Part model, mm, in its own coordinate system. Face numbers are marked on the shaded views. A direction names the side the tool comes from. Give positions to 0.01 mm unless a question says otherwise; leave off trailing zeros. Order: outer loops, then holes, each group sorted by start corner. A loop starts at its lowest first (then second) coordinate and runs counter-clockwise, first axis right, second up. Notation, with made-up numbers: M -35.5,71.5 L -18.5,71.5 A15 cw -18.5,97.5 Z; hole C 7,49.5 d2. An arc over 180 degrees is marked long. Write each question's results on one line, items separated by ' | '. Start each with the question number.
from build123d import *

# Parameters (mm, degrees)
SKETCH_1_R               = 222
EXTRUDE_1_DEPTH          = 76.4
EXTRUDE_2_DEPTH          = 76.4
CUT_EXTRUDE_1_DEPTH      = 508.563749691
CUT_EXTRUDE_1_DEPTH_BACK = 508.563749691
SKETCH_3_R               = 220.4
CUT_EXTRUDE_2_DEPTH      = 508.563749691
CUT_EXTRUDE_2_DEPTH_BACK = 508.563749691
SKETCH_5_R               = 222
EXTRUDE_3_DEPTH          = 1.6
EXTRUDE_4_DEPTH          = 1.6
CUT_EXTRUDE_3_DEPTH      = 508.807049971
CUT_EXTRUDE_3_DEPTH_BACK = 508.807049971
SKETCH_7_R               = 205
SKETCH_8_W               = 25
SKETCH_8_H               = 320
EXTRUDE_5_DEPTH          = 1.6
SKETCH_9_W               = 3.2
SKETCH_9_H               = 20
EXTRUDE_6_DEPTH          = 50
EXTRUDE_7_DEPTH          = 73
SKETCH_19_W              = 40
SKETCH_19_H              = 4
SKETCH_21_R              = 4
CUT_EXTRUDE_5_DEPTH      = 62
CUT_EXTRUDE_6_DEPTH      = 240


with BuildPart() as part:
    # ｽｹｯﾁ1 → ﾎﾞｽ - 押し出し1 (new body)
    with BuildSketch(Plane.XY.offset(1.6)):
        Circle(SKETCH_1_R)
    extrude(amount=EXTRUDE_1_DEPTH)

    # ｽｹｯﾁ2 → ﾎﾞｽ - 押し出し2 (add)
    with BuildSketch(Plane.XY.offset(1.6)):
        Polygon((17.508293028, 221.308516951), (450, 187.092971873), (450, -187.092971873), (17.508293028, -221.308516951), align=None)
    extrude(amount=EXTRUDE_2_DEPTH)

    # ｽｹｯﾁ3 → ｶｯﾄ - 押し出し1 (cut, two sides: drawn at the far end of the back side and taken through both)
    with BuildSketch(Plane.XY.offset(1.6).offset(-CUT_EXTRUDE_1_DEPTH_BACK)):
        Circle(SKETCH_3_R)
    extrude(amount=CUT_EXTRUDE_1_DEPTH + CUT_EXTRUDE_1_DEPTH_BACK, mode=Mode.SUBTRACT)

    # ｽｹｯﾁ4 → ｶｯﾄ - 押し出し2 (cut, two sides: drawn at the far end of the back side and taken through both)
    with BuildSketch(Plane.XY.offset(1.6).offset(-CUT_EXTRUDE_2_DEPTH_BACK)):
        Polygon((17.382107132, 219.713500613), (448.4, 185.614552806), (448.4, -185.614552806), (17.382107132, -219.713500613), align=None)
    extrude(amount=CUT_EXTRUDE_2_DEPTH + CUT_EXTRUDE_2_DEPTH_BACK, mode=Mode.SUBTRACT)

    # ｽｹｯﾁ5 → ﾎﾞｽ - 押し出し3 (add)
    with BuildSketch(Plane.XY):
        with Locations(Location((0, 0, 0), (0, 0, 274.523396987))):
            Circle(SKETCH_5_R)
    extrude(amount=EXTRUDE_3_DEPTH)

    # ｽｹｯﾁ6 → ﾎﾞｽ - 押し出し4 (add)
    with BuildSketch(Plane.XY):
        Polygon((17.508293028, 221.308516951), (450, 187.092971873), (450, -187.092971873), (17.508293028, -221.308516951), align=None)
    extrude(amount=EXTRUDE_4_DEPTH)

    # ｽｹｯﾁ7 → ｶｯﾄ - 押し出し3 (cut, two sides: drawn at the far end of the back side and taken through both)
    with BuildSketch(Plane.XY.offset(-CUT_EXTRUDE_3_DEPTH_BACK)):
        Circle(SKETCH_7_R)
    extrude(amount=CUT_EXTRUDE_3_DEPTH + CUT_EXTRUDE_3_DEPTH_BACK, mode=Mode.SUBTRACT)

    # ｽｹｯﾁ8 → ﾎﾞｽ - 押し出し5 (add)
    with BuildSketch(Plane.XY.offset(60.4)):
        with Locations((462.5, 0)):
            Rectangle(SKETCH_8_W, SKETCH_8_H)
    extrude(amount=EXTRUDE_5_DEPTH)

    # ｽｹｯﾁ9 → ﾎﾞｽ - 押し出し6 (add)
    with BuildSketch(Plane.XY):
        with Locations((451.6, 0)):
            Rectangle(SKETCH_9_W, SKETCH_9_H)
    extrude(amount=EXTRUDE_6_DEPTH)

    # ｽｹｯﾁ10 → ﾎﾞｽ - 押し出し7 (add)
    with BuildSketch(Plane.XY.offset(5)):
        with BuildLine():
            Line((9.925134298, 221.778023504), (10.068199297, 224.974823842))
            ThreePointArc((10.068199297, 224.974823842), (0, 225.2), (-10.068199297, 224.974823842))
            Line((-10.068199297, 224.974823842), (-9.925134298, 221.778023504))
            ThreePointArc((-9.925134298, 221.778023504), (0, 222), (9.925134298, 221.778023504))
        make_face()
    extrude(amount=EXTRUDE_7_DEPTH)

    # ｽｹｯﾁ11 → ｶｯﾄ - 回転1 (revolve, cut)
    with BuildSketch(Plane.XY.offset(70), mode=Mode.PRIVATE) as cut_revolve_1_sk:
        Polygon((-22.73960217, 199.910856366), (-27.26039783, 239.654565386), (-31.234768732, 239.20248582), (-26.713973072, 199.4587768), align=None)
    revolve(cut_revolve_1_sk.sketch.rotate(Axis((-22.73960217, 199.910856366, 70), (-0.11301989150090416, 0.9935927254791693, 0)), 180), axis=Axis((-22.73960217, 199.910856366, 70), (-0.11301989150090416, 0.9935927254791693, 0)), mode=Mode.SUBTRACT)

    # ｽｹｯﾁ12 → ｶｯﾄ - 回転2 (revolve, cut)
    with BuildSketch(Plane.XY.offset(70), mode=Mode.PRIVATE) as cut_revolve_2_sk:
        Polygon((23.422676304, 199.975624659), (26.577323696, 239.851033119), (22.58978285, 240.166497858), (19.435135458, 200.291089398), align=None)
    revolve(cut_revolve_2_sk.sketch.rotate(Axis((23.422676304, 199.975624659, 70), (0.07886618481164225, 0.996885211492906, 0)), 180), axis=Axis((23.422676304, 199.975624659, 70), (0.07886618481164225, 0.996885211492906, 0)), mode=Mode.SUBTRACT)

    # ｽｹｯﾁ13 → ｶｯﾄ - 回転3 (revolve, cut)
    with BuildSketch(Plane.XY.offset(70), mode=Mode.PRIVATE) as cut_revolve_3_sk:
        Polygon((193.422676304, 186.526482006), (196.577323696, 226.401890466), (192.58978285, 226.717355205), (189.435135458, 186.841946746), align=None)
    revolve(cut_revolve_3_sk.sketch.rotate(Axis((193.422676304, 186.526482006, 70), (0.078866184811642, 0.9968852114929061, 0)), 180), axis=Axis((193.422676304, 186.526482006, 70), (0.078866184811642, 0.9968852114929061, 0)), mode=Mode.SUBTRACT)

    # ｽｹｯﾁ14 → ｶｯﾄ - 回転4 (revolve, cut)
    with BuildSketch(Plane.XY.offset(70), mode=Mode.PRIVATE) as cut_revolve_4_sk:
        Polygon((433.422676304, 167.539457084), (436.577323696, 207.414865544), (432.58978285, 207.730330283), (429.435135458, 167.854921824), align=None)
    revolve(cut_revolve_4_sk.sketch.rotate(Axis((433.422676304, 167.539457084, 70), (0.07886618481164205, 0.9968852114929061, 0)), 180), axis=Axis((433.422676304, 167.539457084, 70), (0.07886618481164205, 0.9968852114929061, 0)), mode=Mode.SUBTRACT)

    # ｽｹｯﾁ15 → ｶｯﾄ - 回転5 (revolve, cut)
    with BuildSketch(Plane.XY.offset(70), mode=Mode.PRIVATE) as cut_revolve_5_sk:
        Polygon((-22.73960217, -199.910856366), (-27.26039783, -239.654565386), (-23.286026928, -240.106644952), (-18.765231268, -200.362935932), align=None)
    revolve(cut_revolve_5_sk.sketch.rotate(Axis((-22.73960217, -199.910856366, 70), (-0.11301989150090416, -0.9935927254791693, 0)), 180), axis=Axis((-22.73960217, -199.910856366, 70), (-0.11301989150090416, -0.9935927254791693, 0)), mode=Mode.SUBTRACT)

    # ｽｹｯﾁ16 → ｶｯﾄ - 回転6 (revolve, cut)
    with BuildSketch(Plane.XY.offset(70), mode=Mode.PRIVATE) as cut_revolve_6_sk:
        Polygon((23.422676304, -199.975624659), (26.577323696, -239.851033119), (30.564864542, -239.53556838), (27.41021715, -199.66015992), align=None)
    revolve(cut_revolve_6_sk.sketch.rotate(Axis((23.422676304, -199.975624659, 70), (0.07886618481164225, -0.996885211492906, 0)), 180), axis=Axis((23.422676304, -199.975624659, 70), (0.07886618481164225, -0.996885211492906, 0)), mode=Mode.SUBTRACT)

    # ｽｹｯﾁ17 → ｶｯﾄ - 回転7 (revolve, cut)
    with BuildSketch(Plane.XY.offset(70), mode=Mode.PRIVATE) as cut_revolve_7_sk:
        Polygon((193.422676304, -186.526482006), (196.577323696, -226.401890466), (200.564864542, -226.086425727), (197.41021715, -186.211017267), align=None)
    revolve(cut_revolve_7_sk.sketch.rotate(Axis((193.422676304, -186.526482006, 70), (0.078866184811642, -0.9968852114929061, 0)), 180), axis=Axis((193.422676304, -186.526482006, 70), (0.078866184811642, -0.9968852114929061, 0)), mode=Mode.SUBTRACT)

    # ｽｹｯﾁ18 → ｶｯﾄ - 回転8 (revolve, cut)
    with BuildSketch(Plane.XY.offset(70), mode=Mode.PRIVATE) as cut_revolve_8_sk:
        Polygon((433.422676304, -167.539457084), (436.577323696, -207.414865544), (440.564864542, -207.099400805), (437.41021715, -167.223992345), align=None)
    revolve(cut_revolve_8_sk.sketch.rotate(Axis((433.422676304, -167.539457084, 70), (0.07886618481164205, -0.9968852114929061, 0)), 180), axis=Axis((433.422676304, -167.539457084, 70), (0.07886618481164205, -0.9968852114929061, 0)), mode=Mode.SUBTRACT)

    # ｽｹｯﾁ19 → ｶｯﾄ - 回転9 (revolve, cut)
    with BuildSketch(Plane.XY.offset(70), mode=Mode.PRIVATE) as cut_revolve_9_sk:
        with Locations((-221.2, -2)):
            Rectangle(SKETCH_19_W, SKETCH_19_H)
    revolve(cut_revolve_9_sk.sketch.rotate(Axis((-201.2, 0, 70), (-1, 0, 0)), 270), axis=Axis((-201.2, 0, 70), (-1, 0, 0)), mode=Mode.SUBTRACT)

    # ｽｹｯﾁ21 → ｶｯﾄ - 押し出し5 (cut)
    with BuildSketch(Plane.XY):
        with Locations((465, -150)):
            Circle(SKETCH_21_R)
        with Locations((465, -15)):
            Circle(SKETCH_21_R)
        with Locations((465, 15)):
            Circle(SKETCH_21_R)
        with Locations((465, 150)):
            Circle(SKETCH_21_R)
    extrude(amount=CUT_EXTRUDE_5_DEPTH, mode=Mode.SUBTRACT)

    # ｽｹｯﾁ22 → ｶｯﾄ - 押し出し6 (cut)
    with BuildSketch(Plane(origin=(0, 0, 0), x_dir=(1, 0, 0), z_dir=(0, 1, 0))):
        with BuildLine():
            Line((-35, -56), (35, -56))
            ThreePointArc((35, -56), (42.071067812, -53.071067812), (45, -46))
            Line((45, -46), (45, -21))
            ThreePointArc((45, -21), (42.071067812, -13.928932188), (35, -11))
            Line((35, -11), (-35, -11))
            ThreePointArc((-35, -11), (-42.071067812, -13.928932188), (-45, -21))
            Line((-45, -21), (-45, -46))
            ThreePointArc((-45, -46), (-42.071067812, -53.071067812), (-35, -56))
        make_face()
    extrude(amount=-CUT_EXTRUDE_6_DEPTH, mode=Mode.SUBTRACT)

    # ｽｹｯﾁ23 → ｶｯﾄ - 回転10 (revolve, cut)
    with BuildSketch(Plane.XY.offset(33.5), mode=Mode.PRIVATE) as cut_revolve_10_sk:
        Polygon((-50.027124774, -194.881314617), (-59.972875226, -233.62511474), (-57.93882572, -234.147266638), (-47.993075268, -195.403466516), align=None)
    revolve(cut_revolve_10_sk.sketch.rotate(Axis((-50.027124774, -194.881314617, 33.5), (-0.24864376130198912, -0.9685950030666065, 0)), 180), axis=Axis((-50.027124774, -194.881314617, 33.5), (-0.24864376130198912, -0.9685950030666065, 0)), mode=Mode.SUBTRACT)

    # ｽｹｯﾁ24 → ｶｯﾄ - 回転11 (revolve, cut)
    with BuildSketch(Plane.XY.offset(33.5), mode=Mode.PRIVATE) as cut_revolve_11_sk:
        Polygon((53.422676304, -197.602246544), (56.577323696, -237.477655004), (58.67078264, -237.312036016), (55.516135248, -197.436627556), align=None)
    revolve(cut_revolve_11_sk.sketch.rotate(Axis((53.422676304, -197.602246544, 33.5), (0.07886618481164233, -0.996885211492906, 0)), 180), axis=Axis((53.422676304, -197.602246544, 33.5), (0.07886618481164233, -0.996885211492906, 0)), mode=Mode.SUBTRACT)


solid = part.part
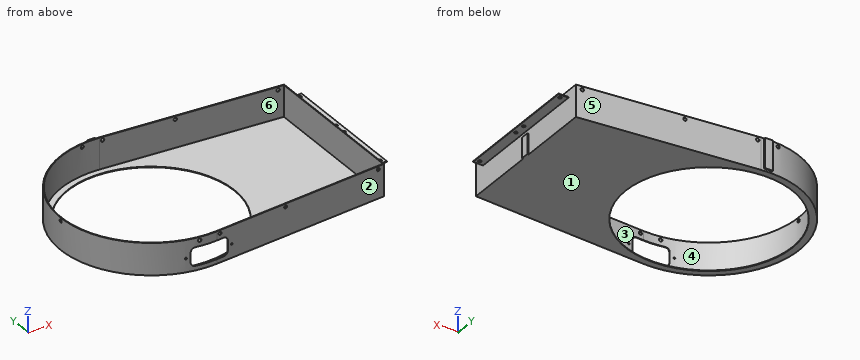
(1) Pull direction X, two halves, no side cores. Call the marked faces 1, 2, 3 and 4: +X half, -X half, draft (parallel to the pull), parting line (faces both ways), or undercut.
(2) Probe L1, parallel to X at y = 15, z = 61; L2, parallel to Y at x = 465, z = 61.3; L3, parallel to X at y = 5, z = 33. List the from-to ranges inside material, lowest first.
(3) Tool access for the marked faces 5 and 6: list every direction of +Z, -Z, +X, -X, +Y, -Y with a clear straight run to the whole face (end or side of a thin tool).
(4) Saw through at D-D on x = 247.5. Give the cut face in (y, z), plus the area to 3 significant figures.
(5) Drop flat-ended pins along their axis: P1, Ø12, axis at y = -28.5, z = 49.5, coming from the -X side; P2, Ø22, axis at y = 3, z = 21.5, coming from the +X side; P3, Ø2.5, axis at x = 452, z = 32, coming from the -Y side. Give the stop position or say it passes through.
(6) Saw through at C-C on x = 163. Give the cut face in (y, z).
(7) Saw through at A-A on x = 0. Give the cut face in (y, z).
(8) Saw through at B-B on y = -102. Give the cut face in (x, z), plus the area to 3 significant figures.
Taken from the geometry:
1) face 1: draft | face 2: +X half | face 3: undercut | face 4: undercut
2) L1: x = -221.49 to -219.89, 448.4 to 461, 469 to 475 | L2: y = -160 to -154, -146 to -19, -11 to 11, 19 to 146, 154 to 160 | L3: x = -221.94 to -220.34, 448.4 to 453.2
3) face 5: +Z, -Z, +X, +Y | face 6: +Z
4) outline: M -203.11,0 L 203.11,0 L 203.11,78 L 201.51,78 L 201.51,1.6 L -201.51,1.6 L -201.51,78 L -203.11,78 Z | area: 895 mm²
5) P1: stops at x = -220.86 | P2: stops at x = 453.2 | P3: stops at y = -10
6) outline: M -209.8,0 L -124.32,0 L -124.32,1.6 L -208.19,1.6 L -208.19,78 L -209.8,78 Z; M 124.32,0 L 209.8,0 L 209.8,78 L 208.19,78 L 208.19,1.6 L 124.32,1.6 Z
7) outline: M -222,0 L -205,0 L -205,1.6 L -220.4,1.6 L -220.4,11 L -222,11 Z; M -222,56 L -220.4,56 L -220.4,78 L -222,78 Z; M 205,0 L 222,0 L 222,5 L 225.2,5 L 225.2,78 L 220.4,78 L 220.4,1.6 L 205,1.6 Z
8) outline: M -197.18,0 L -177.82,0 L -177.82,1.6 L -195.38,1.6 L -195.38,78 L -197.18,78 Z; M 177.82,0 L 450,0 L 450,60.4 L 475,60.4 L 475,62 L 450,62 L 450,78 L 448.4,78 L 448.4,1.6 L 177.82,1.6 Z | area: 766 mm²
